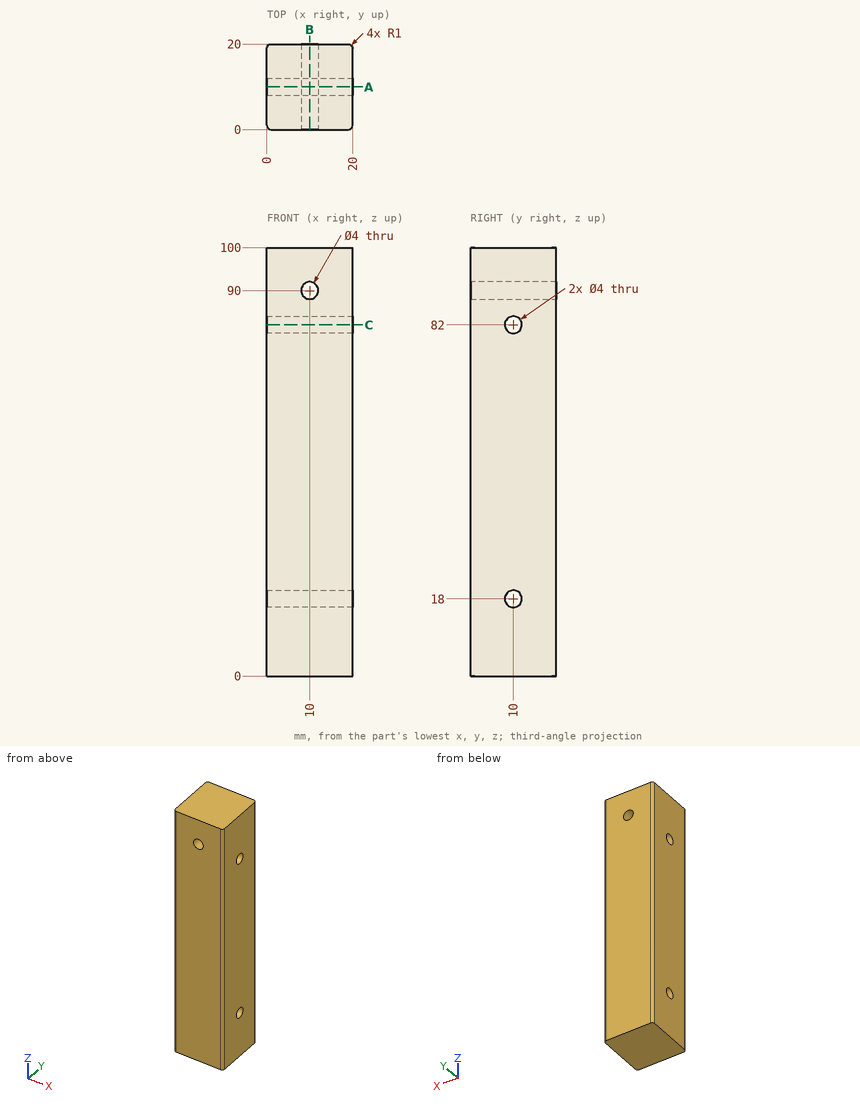
Here's the drawing with two shaded views (mm, measured from the low corner). I have some questions. Coordinates: 2 decimals unless noted, no trailing zeros. Loops run counter-clockwise (first coordinate to the right, second up) from the corner with the lowest first, then second, coordinate; pieces in that order, holes last. Notation, with made-up numbers: M -36,58 L -23,58 A26 cw -23,96 Z; hole C -34,64.25 d10. An arc over 180 degrees is marked long. Put each result on its own line as item: value. Start each with the question number.
(1) Imagine slicing it at A-A on y = 10. List the corners of the cut face in (x, z) for me, and give its area (3 significant figures).
(2) Imagine slicing it at C-C on z = 82. List the corners of the cut face in (x, y) for me, and give its area (3 significant figures).
(3) Imagine slicing it at B-B on x = 10. List the corners of the cut face in (y, z) for me, and give its area (3 significant figures).
(4) I need wall thicknesses on probe 1 along Y at (x, z) = (15.75, 18); probe 2 along Z at (x, y) = (11.75, 9.25). Which ranges of each line are inside material? Lowest first, please.
Worked answers:
1. outline: M 0,0 L 20,0 L 20,16 L 0,16 Z; M 0,20 L 20,20 L 20,80 L 0,80 Z; M 0,84 L 20,84 L 20,100 L 0,100 Z; hole C 10,90 d4
1. area: 1,830 mm2
2. outline: M 0,1 A1 ccw 1,0 L 19,0 A1 ccw 20,1 L 20,8 L 0,8 Z; M 0,12 L 20,12 L 20,19 A1 ccw 19,20 L 1,20 A1 ccw 0,19 Z
2. area: 319 mm2
3. outline: M 0,0 L 20,0 L 20,88 L 0,88 Z; M 0,92 L 20,92 L 20,100 L 0,100 Z; hole C 10,18 d4; hole C 10,82 d4
3. area: 1,890 mm2
4. probe 1: y = 0 to 8, 12 to 20
4. probe 2: z = 0 to 16.15, 19.85 to 80.15, 83.85 to 89.03, 90.97 to 100
